```python
from build123d import *

# Parameters (mm, degrees)
BOSS_EXTRU_2_DEPTH      = 3
ESQUISSE2_R             = 3.25
ENL_V_MAT_EXTRU_1_DEPTH = 10


with BuildPart() as part:
    # Esquisse1 → Boss.-Extru.2 (new body)
    with BuildSketch(Plane.XY):
        with BuildLine():
            ThreePointArc((-12.288149304, -10.247018429), (0.000780623, -15.999999981), (12.289149128, -10.245819328))
            ThreePointArc((12.289149128, -10.245819328), (9.309773091, -5.375), (15.017714385, -5.519805672))
            ThreePointArc((15.017714385, -5.519805672), (13.856406461, 8), (2.728565257, 15.765625))
            ThreePointArc((2.728565257, 15.765625), (0, 10.75), (-2.728565257, 15.765625))
            ThreePointArc((-2.728565257, 15.765625), (-13.856384318, 8.000038352), (-15.01774494, -5.519722539))
            ThreePointArc((-15.01774494, -5.519722539), (-9.310492225, -5.375986513), (-12.288149304, -10.247018429))
        make_face()
    extrude(amount=BOSS_EXTRU_2_DEPTH)

    # Esquisse2 → Enlèv. mat.-Extru.1 (cut)
    with BuildSketch(Plane.XY.offset(3)):
        with Locations((-9.309773091, 5.375)):
            Circle(ESQUISSE2_R)
        with Locations((9.309773091, 5.375)):
            Circle(ESQUISSE2_R)
        with Locations((0, -10.75)):
            Circle(ESQUISSE2_R)
    extrude(amount=-ENL_V_MAT_EXTRU_1_DEPTH, mode=Mode.SUBTRACT)


solid = part.part
```
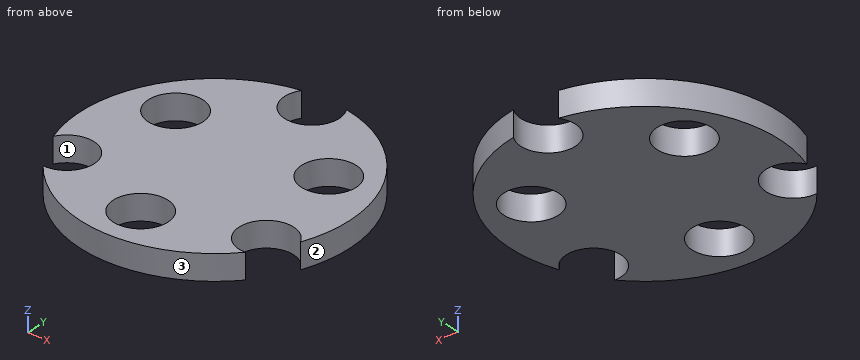
Geometry check sheet. Reference: the model listing, model coordinates, mm. Face numbers are marked on the shaded views. Round coordinates to 2 decimals unless told otherwise and drop trailing zeros. Order: outer loops, then holes, each group sorted by start corner. A loop starts at its lowest first (then second) coordinate and runs counter-clockwise, first axis right, second up. Notation, with made-up numbers: (-28.5, 73) - (6.5, 73) arc R26 ccw to (6.5, 104) - close; hole circle Ø11 at (-28, 32.5). An arc over 180 degrees is marked (long way). Use a Markdown table: item, result. Add a question column.
(1) Depth check by flat-ended pin: pin 1 (1.5 mm diameter, centred on y = -10.5, z = 1, fed in from -X); pin 2 (4 mm diameter, centred on x = 9.31, y = 5.38, fed in from +Z). Enter the tip coordinate at first touch or a pass-through.
(2) Sectioned sample at D-D, the plane x = 10. Enter the section's corners in (y, z), and give its area (3 significant figures).
(3) Sectioned sample at A-A, the plane x = 0. Enter the section's corners in (y, z), and give its area (4 significant figures).
(4) Sectioned sample at C-C, the plane z = 1.3. Enter the section's corners in (x, y) (3 decimals), and give its area (3 significant figures).
(5) Material ranges on line 1 along Y through (x, z) = (3, 0.45); line 2 along X through (y, z) = (-0.5, 2.45); line 3 along Y through (x, z) = (7.5, 0.75), recorded low to high. Write a range as [from, to].
(6) Sectioned sample at B-B, the plane y = -12. Enter the section's corners in (x, z), and give its area (3 significant figures).
(7) Release check for a two-part mould opening along X. For the marked faces 1, 2 and 3 record: pulls with the +X half, pulls with the -X half, needs draft (parallel to the pull), parting line crosses it, or undercut.
Answers below:
| question | item | result |
|---|---|---|
| 1 | pin 1 | x = -12.29 |
| 1 | pin 2 | through |
| 2 | outline | (-12.49, 0) - (-9.46, 0) - (-9.46, 3) - (-12.49, 3) - close; (-4.54, 0) - (2.2, 0) - (2.2, 3) - (-4.54, 3) - close; (8.55, 0) - (12.49, 0) - (12.49, 3) - (8.55, 3) - close |
| 2 | area | 41.1 mm² |
| 3 | outline | (-16, 0) - (-14, 0) - (-14, 3) - (-16, 3) - close; (-7.5, 0) - (10.75, 0) - (10.75, 3) - (-7.5, 3) - close |
| 3 | area | 60.75 mm² |
| 4 | outline | (-15.018, -5.52) arc R3.25 cw (long way) to (-12.288, -10.247) arc R16 ccw to (12.289, -10.246) arc R3.25 cw (long way) to (15.018, -5.52) arc R16 ccw to (2.729, 15.766) arc R3.25 cw (long way) to (-2.729, 15.766) arc R16 ccw to start; hole circle Ø6.5 at (-9.31, 5.375); hole circle Ø6.5 at (0, -10.75); hole circle Ø6.5 at (9.31, 5.375) |
| 4 | area | 620 mm² |
| 5 | line 1 | [-15.72, -12], [-9.5, 12.75], [15.25, 15.72] |
| 5 | line 2 | [-15.99, 15.99] |
| 5 | line 3 | [-14.13, 2.68], [8.07, 14.13] |
| 6 | outline | (-10.58, 0) - (-3, 0) - (-3, 3) - (-10.58, 3) - close; (3, 0) - (10.58, 0) - (10.58, 3) - (3, 3) - close |
| 6 | area | 45.5 mm² |
| 7 | face 1 | undercut |
| 7 | face 2 | pulls with the +X half |
| 7 | face 3 | parting line crosses it |
